```python
from build123d import *

# Parameters (mm, degrees)
SKETCH3_W           = 26
SKETCH3_H           = 25
BOSS_EXTRUDE2_DEPTH = 22
SKETCH4_R           = 5
BOSS_EXTRUDE3_DEPTH = 1
SKETCH5_R           = 4
BOSS_EXTRUDE4_DEPTH = 9
SKETCH7_W           = 8
SKETCH7_H           = 2.6
CUT_EXTRUDE1_DEPTH  = 5
SKETCH8_R           = 1.5
CUT_EXTRUDE2_DEPTH  = 6


with BuildPart() as part:
    # Sketch3 → Boss-Extrude2 (new body)
    with BuildSketch(Plane.XY):
        Rectangle(SKETCH3_W, SKETCH3_H)
    extrude(amount=BOSS_EXTRUDE2_DEPTH)

    # Sketch4 → Boss-Extrude3 (add)
    with BuildSketch(Plane(origin=(13, 0, 0), x_dir=(0, 0, -1), z_dir=(1, 0, 0))):
        with Locations((-11.15653954, 0)):
            Circle(SKETCH4_R)
    extrude(amount=BOSS_EXTRUDE3_DEPTH)

    # Sketch5 → Boss-Extrude4 (add)
    with BuildSketch(Plane(origin=(14, 0, 0), x_dir=(0, 0, -1), z_dir=(1, 0, 0))):
        with Locations((-11.15653954, 0)):
            Circle(SKETCH5_R)
    extrude(amount=BOSS_EXTRUDE4_DEPTH)

    # Sketch7 → Cut-Extrude1 (cut)
    with BuildSketch(Plane.XY.offset(11)):
        with Locations((19, 0)):
            Rectangle(SKETCH7_W, SKETCH7_H)
    cut_extrude1 = extrude(amount=-CUT_EXTRUDE1_DEPTH, mode=Mode.SUBTRACT)

    # Mirror1: Cut-Extrude1 across plane
    add(cut_extrude1.mirror(Plane.XY.offset(11)), mode=Mode.SUBTRACT)

    # Sketch8 → Cut-Extrude2 (cut)
    with BuildSketch(Plane(origin=(0, 0, 0), x_dir=(1, 0, 0), z_dir=(0, 1, 0))):
        with Locations(Location((19, -11, 0), (0, 0, 270))):
            Circle(SKETCH8_R)
    cut_extrude2 = extrude(amount=-CUT_EXTRUDE2_DEPTH, mode=Mode.SUBTRACT)

    # Mirror2: Cut-Extrude2 across plane
    add(cut_extrude2.mirror(Plane.ZX), mode=Mode.SUBTRACT)


solid = part.part
```
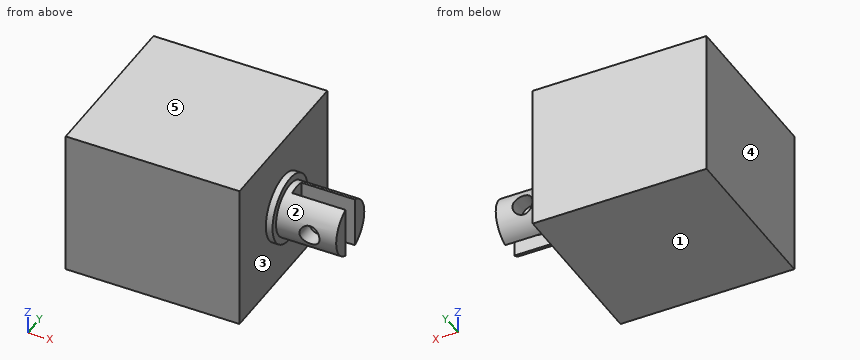
Verification items for the finished model (mm, model axes). Face numbers are marked on the shaded views. A direction names the side the tool comes from. Coordinates: 2 decimals unless noted, no trailing zeros. Loops run counter-clockwise (first coordinate to the right, second up) from the corner with the lowest first, then second, coordinate; pieces in that order, holes last. Notation, with made-up numbers: (51, -10) -> (59, -10) arc R12 cw to (59, 6) -> close; hole circle Ø9 at (89, 73.5). An arc over 180 degrees is marked (long way). Answer in a Markdown table with one row per item. Add a question column.
1. Section check D-D, the plane z = 5.5. Enter the section's corners in (x, y), then the cut area to 3 significant figures.
2. Draft check along X on the marked faces 3, 4 and 5. Enter one of: +X half, -X half, draft (parallel to the pull), parting line (faces both ways), or undercut.
3. Section check C-C, the plane x = 19. Enter the section's corners in (y, z).
4. Depth check by flat-ended pin: P1, Ø5, axis at x = 19, z = 11, coming from the +Y side; P2, Ø1.3, axis at y = -0.5, z = 11, coming from the +X side; P3, Ø10, axis at x = 18.5, z = 8.5, coming from the -Y side; P4, Ø2.5, axis at x = 19, z = 11, coming from the +Y side. Enter the tip coordinate at first touch or a pass-through.
5. Material ranges on probe 1 along X at (y, z) = (-3, 11); probe 2 along Z at (x, y) = (19, 2.4); probe 3 along Z at (x, y) = (19, -2.6), recorded low to high. Write a range as [from, to].
6. Access from +Z, -Z, +X, -X, +Y, -Y to the whole of each face (thin tool, end or side, straight path). Record for the marked faces 1 and 2.
7. Section check B-B, the plane z = 11. Enter the section's corners in (x, y).
8. Section check A-A, the plane y = 0. Enter the section's corners in (x, z), then the cut area to 3 significant figures.
Derived:
| question | item | result |
|---|---|---|
| 1 | outline | (-13, -12.5) -> (13, -12.5) -> (13, 12.5) -> (-13, 12.5) -> close |
| 1 | area | 650 mm² |
| 2 | face 3 | +X half |
| 2 | face 4 | -X half |
| 2 | face 5 | draft |
| 3 | outline | (-3.77, 12.5) -> (-1.3, 12.5) -> (-1.3, 14.94) arc R4 ccw to start; (-3.64, 9.5) arc R4 ccw to (-1.3, 7.37) -> (-1.3, 9.5) -> close; (1.3, 7.37) arc R4 ccw to (3.64, 9.5) -> (1.3, 9.5) -> close; (1.3, 12.5) -> (3.77, 12.5) arc R4 ccw to (1.3, 14.94) -> close |
| 4 | P1 | stops at y = 4 |
| 4 | P2 | stops at x = 15 |
| 4 | P3 | stops at y = -4.98 |
| 4 | P4 | passes through |
| 5 | probe 1 | x = [-13, 17.5], [20.5, 23] |
| 5 | probe 2 | z = [7.96, 9.5], [12.5, 14.36] |
| 5 | probe 3 | z = [8.12, 9.5], [12.5, 14.2] |
| 6 | face 1 | -Z, +X, -X, +Y, -Y |
| 6 | face 2 | +X |
| 7 | outline | (-13, -12.5) -> (13, -12.5) -> (13, -5) -> (14, -5) -> (14, -4) -> (17.5, -4) -> (17.5, -1.3) -> (15, -1.3) -> (15, 1.3) -> (17.5, 1.3) -> (17.5, 4) -> (14, 4) -> (14, 5) -> (13, 5) -> (13, 12.5) -> (-13, 12.5) -> close; (20.5, -4) -> (23, -4) -> (23, -1.3) -> (20.5, -1.3) -> close; (20.5, 1.3) -> (23, 1.3) -> (23, 4) -> (20.5, 4) -> close |
| 8 | outline | (-13, 0) -> (13, 0) -> (13, 6.16) -> (14, 6.16) -> (14, 7.16) -> (15, 7.16) -> (15, 15.16) -> (14, 15.16) -> (14, 16.16) -> (13, 16.16) -> (13, 22) -> (-13, 22) -> close |
| 8 | area | 590 mm² |
